Could you check a few things on this model? Use its own coordinates, in mm. A direction names the side the tool comes from. Coordinates: 2 decimals unless noted, no trailing zeros. Loops run counter-clockwise (first coordinate to the right, second up) from the corner with the lowest first, then second, coordinate; pieces in that order, holes last.
from build123d import *

# Parameters (mm, degrees)
F0_W          = 76.2
F0_H          = 38.1
F1_DEPTH      = 25.4
F3_R          = 3.81
F4_DEPTH      = 25.4
F5_R          = 11.0802185983
F6_DEPTH      = 38.1
F2_R          = 3.81
F7_DEPTH      = 25.4
F8_R          = 3.81
F9_DEPTH      = 25.4
F11_R         = 3.81
F12_DEPTH     = 25.4
F10_W         = 12.7
F10_H         = 12.7
F14_R         = 2.54
F15_R         = 2.54
F17_T1_DEPTH  = 29.21
F17_S5_W      = 2.54
F17_S5_H      = 2.54
F17_T6_DEPTH  = 2.54
F17_S11_W     = 2.54
F17_S11_H     = 2.54
F17_T12_DEPTH = 2.54


# Not quite as in the source:
# - a fillet or chamfer that OpenCascade refuses, or shapes differently, is made with other operations: its cross-section is extruded or revolved along the edge and cut away or added


with BuildPart() as f1:
    # F0 (on Top) → F1 (new body)
    with BuildSketch(Plane.XY):
        with Locations((2.4286340922, -4.9461158044)):
            Rectangle(F0_W, F0_H)
    extrude(amount=F1_DEPTH)

    # F3 (on face) → F4 (cut)
    with BuildSketch(Plane.XY.offset(25.4)):
        with Locations((32.9086340922, 6.4838841956)):
            Circle(F3_R)
    extrude(amount=-F4_DEPTH, mode=Mode.SUBTRACT)

    # F5 (on face) → F6 (join)
    with BuildSketch(Plane.XY.offset(25.4)):
        with Locations((2.4286331609, -4.0792874061)):
            Circle(F5_R)
    extrude(amount=F6_DEPTH)

    # F2 (on face) → F7 (cut)
    with BuildSketch(Plane.XY.offset(25.4)):
        with Locations((-28.0513659078, 6.4838841956)):
            Circle(F2_R)
    extrude(amount=-F7_DEPTH, mode=Mode.SUBTRACT)

    # F8 (on face) → F9 (cut)
    with BuildSketch(Plane.XY.offset(25.4)):
        with Locations((-28.0513659078, -16.3761158044)):
            Circle(F8_R)
    extrude(amount=-F9_DEPTH, mode=Mode.SUBTRACT)

    # F11 (on face) → F12 (cut)
    with BuildSketch(Plane.XY.offset(25.4)):
        with Locations((32.9086340922, -16.3761158044)):
            Circle(F11_R)
    extrude(amount=-F12_DEPTH, mode=Mode.SUBTRACT)

    # F10 (on Front) → F13 (revolve, cut)
    with BuildSketch(Plane.XZ):
        with Locations((-10.6504372485, 48.6334538215)):
            Rectangle(F10_W, F10_H)
    revolve(axis=Axis((2.4286331609, -4.0792874061, 25.4), (0, 0, -1)), mode=Mode.SUBTRACT)

    # F14
    f14_edges = [f1.edges().sort_by_distance(p)[0] for p in [
        (2.428634, -23.996116, 25.4),
    ]]
    fillet(f14_edges, radius=F14_R)

    # F15
    f15_edges = [f1.edges().sort_by_distance(p)[0] for p in [
        (-35.671366, -3.676116, 25.4),
        (2.428634, 14.103884, 25.4),
        (40.528634, -3.676116, 25.4),
    ]]
    fillet(f15_edges, radius=F15_R)

    # F16: fillet of radius 5.08 on 2 edges, made by hand

    # F16_s1 → F16_t2 (revolve, cut)
    with BuildSketch(Plane.XZ.offset(4.0792874061)):
        with BuildLine():
            ThreePointArc((13.5088517592, 58.42), (12.0209542077, 62.0121024484), (8.4288517592, 63.5))
            Line((8.4288517592, 63.5), (8.4288517592, 63.6016))
            Line((8.4288517592, 63.6016), (13.6104517592, 63.6016))
            Line((13.6104517592, 63.6016), (13.6104517592, 58.42))
            Line((13.6104517592, 58.42), (13.5088517592, 58.42))
        make_face()
    revolve(axis=Axis((2.4286331609, -4.0792874061, 63.5), (0, 0, 1)), mode=Mode.SUBTRACT)

    # F16_s3 → F16_t4 (revolve, cut)
    with BuildSketch(Plane.XZ.offset(4.0792874061)):
        with BuildLine():
            ThreePointArc((13.5088517592, 37.5596735125), (12.630027146, 40.4156366371), (10.2976212989, 42.2834538215))
            Line((10.2976212989, 42.2834538215), (10.3349966897, 42.3779294277))
            ThreePointArc((10.3349966897, 42.3779294277), (11.9032365291, 42.3850538215), (13.5088517592, 42.3850538215))
            Line((13.5088517592, 42.3850538215), (13.6104517592, 42.2834538215))
            Line((13.6104517592, 42.2834538215), (13.6104517592, 37.5596735125))
            Line((13.6104517592, 37.5596735125), (13.5088517592, 37.5596735125))
        make_face()
    revolve(axis=Axis((2.4286331609, -4.0792874061, 42.2834538215), (0, 0, -1)), mode=Mode.SUBTRACT)

    # F17: fillet of radius 2.54 on 2 edges, made by hand

    # F17_s2 → F17_t1 (cut)
    with BuildSketch(Plane.XY.offset(-6.35)):
        with BuildLine():
            ThreePointArc((-35.6713659078, 11.5638841956), (-34.927417132, 13.3599354199), (-33.1313659078, 14.1038841956))
            Line((-33.1313659078, 14.1038841956), (-35.6713659078, 14.1038841956))
            Line((-35.6713659078, 14.1038841956), (-35.6713659078, 11.5638841956))
        make_face()
        with BuildLine():
            ThreePointArc((40.5286340922, 11.5638841956), (39.7846853164, 13.3599354199), (37.9886340922, 14.1038841956))
            Line((37.9886340922, 14.1038841956), (40.5286340922, 14.1038841956))
            Line((40.5286340922, 14.1038841956), (40.5286340922, 11.5638841956))
        make_face()
    extrude(amount=F17_T1_DEPTH, mode=Mode.SUBTRACT)


with BuildPart() as f17_tool4:
    # F17_s5 → F17_t6 (new body)
    with BuildSketch(Plane.YZ.offset(37.9886340922)):
        with Locations((12.8338841956, 24.13)):
            Rectangle(F17_S5_W, F17_S5_H)
    extrude(amount=F17_T6_DEPTH)

    # F17_s7 → F17_t8 (revolve, cut)
    with BuildSketch(Plane(origin=(37.9886340922, 11.5638841956, 22.86), x_dir=(0, -0.7071067812, -0.7071067812), z_dir=(0, -0.7071067812, 0.7071067812))):
        with BuildLine():
            ThreePointArc((0, -2.54), (2.54, 0), (0, 2.54))
            Line((0, 2.54), (0, -2.54))
        make_face()
    revolve(axis=Axis((37.9886340922, 11.5638841956, 22.86), (1, 0, 0)), mode=Mode.SUBTRACT)


with BuildPart() as f1_1:
    add(f1.part)

    # F17_t3: cut F17_tool4
    add(f17_tool4.part, mode=Mode.SUBTRACT)


with BuildPart() as f17_tool10:
    # F17_s11 → F17_t12 (new body)
    with BuildSketch(Plane.YZ.offset(-33.1313659078)):
        with Locations((12.8338841956, 24.13)):
            Rectangle(F17_S11_W, F17_S11_H)
    extrude(amount=-F17_T12_DEPTH)

    # F17_s13 → F17_t14 (revolve, cut)
    with BuildSketch(Plane(origin=(-33.1313659078, 11.5638841956, 22.86), x_dir=(0, -0.7071067812, -0.7071067812), z_dir=(0, 0.7071067812, -0.7071067812))):
        with BuildLine():
            ThreePointArc((0, -2.54), (2.54, 0), (0, 2.54))
            Line((0, 2.54), (0, -2.54))
        make_face()
    revolve(axis=Axis((-33.1313659078, 11.5638841956, 22.86), (-1, 0, 0)), mode=Mode.SUBTRACT)


with BuildPart() as f1_2:
    add(f1_1.part)

    # F17_t9: cut F17_tool10
    add(f17_tool10.part, mode=Mode.SUBTRACT)


solid = f1_2.part
(1) Which directions (+Z, -Z, +X, -X, +Y, -Y) give clear straight access to the entire face, cutting with the end or side of a thin tool? Please do faces 1 (the face through (12.997, -0.751, 56.678)), 2 (the face through (2, -23.996, 11)), 3 (the face through (9.33, -7.86, 48.72)).
Answers:
face 1: +Z
face 2: +Z, -Z, +X, -X, -Y
face 3: none
(2) I need wall thicknesses on probe 1 along Y at (x, z) = (-31.5, 6); probe 2 along X at (y, z) = (10, 9); probe 3 along Z at (x, y) = (-6, -21.5). Which ranges of each line are inside material? Lowest first, please.
Answers:
probe 1: y = -24 to -18, -14.76 to 4.86, 8.1 to 14.1
probe 2: x = -35.67 to -29.52, -26.58 to 31.44, 34.38 to 40.53
probe 3: z = 0 to 25.4
(3) Imagine slicing it at A-A, the plane x = -30. Write out the boundary of the cut face in (y, z), and give its area (3 significant figures).
Answers:
outline: (-24, 0) - (-19.65, 0) - (-19.65, 25.4) - (-21.46, 25.4) arc R2.54 ccw to (-24, 22.86) - close; (-13.1, 0) - (3.21, 0) - (3.21, 25.4) - (-13.1, 25.4) - close; (9.76, 0) - (14.1, 0) - (14.1, 22.86) arc R2.54 ccw to (11.56, 25.4) - (9.76, 25.4) - close
area: 632 mm2
(4) For pin 1 (12 mm diameter, centred on x = 0.5, z = 39, fed in from +Y); pin 2 (2 mm diameter, centred on x = 13.5, y = 3, fed in from +Z); pin 3 (8 mm diameter, centred on x = -8.5, y = -12.5, fed in from +Z), each with a flat end and sliding along its axis, tell me the tip position at first contact or that it passes through.
Answers:
pin 1: stops at y = 7
pin 2: stops at z = 25.4
pin 3: stops at z = 61.8
(5) We'd pull the mould along Z, two halves only. Please class faces 4 (the face through (2.926, 13.34, 24.676)), 5 (the face through (29.885, -18.694, 12.878)), 6 (the face through (2, -5, 0)), 7 (the face through (2, 4, 54.983)): +Z half, -Z half, draft (parallel to the pull), parting line (faces both ways), or undercut.
Answers:
face 4: +Z half
face 5: draft
face 6: -Z half
face 7: undercut
(6) Imagine slicing it at D-D, the plane z = 35. Write out the boundary of the cut face in (x, y).
Answers:
outline: circle Ø22.16 at (2.43, -4.08)
(7) Imagine slicing it at C-C, the plane x = -16. Write out the boundary of the cut face in (y, z), and give its area (3 significant figures).
Answers:
outline: (-24, 0) - (14.1, 0) - (14.1, 22.86) arc R2.54 ccw to (11.56, 25.4) - (-21.46, 25.4) arc R2.54 ccw to (-24, 22.86) - close
area: 965 mm2
(8) Imagine slicing it at B-B, the plane z = 20.5. Write out the boundary of the cut face in (x, y).
Answers:
outline: (-35.67, -21.46) arc R2.54 ccw to (-33.13, -24) - (37.99, -24) arc R2.54 ccw to (40.53, -21.46) - (40.53, 11.56) arc R2.54 ccw to (37.99, 14.1) - (-33.13, 14.1) arc R2.54 ccw to (-35.67, 11.56) - close; hole circle Ø7.62 at (-28.05, -16.38); hole circle Ø7.62 at (-28.05, 6.48); hole circle Ø7.62 at (32.91, -16.38); hole circle Ø7.62 at (32.91, 6.48)
